Read the model definition and answer for the solid it produces. Units are mm, in the model's axes. A direction names the side the tool comes from. Round coordinates to 2 decimals unless told otherwise and drop trailing zeros. Answer as CSV lines item,"result".
```python
from build123d import *

# Parameters (mm, degrees)
SKETCH_1_R      = 11.25
SKETCH_1_R_2    = 1.5
SKETCH_1_W      = 5
SKETCH_1_H      = 10
EXTRUDE_1_DEPTH = 5


with BuildPart() as part:
    # 草图1 → 凸台-拉伸1 (new body)
    with BuildSketch(Plane(origin=(0, 0, 0), x_dir=(1, 0, 0), z_dir=(0, 1, 0))):
        Polygon((0, 0), (180, 0), (180, 5), (185, 5), (185, 15), (180, 15), (180, 19.659044965), (177.85, 19.659044965), (177.85, 18.15), (175.15, 18.15), (175.15, 19.659044965), (172, 19.659044965), (172, 22.65), (175.15, 22.65), (175.15, 24.15), (177.85, 24.15), (177.85, 22.65), (180, 22.65), (180, 27.3), (185, 27.3), (185, 37.3), (180, 37.3), (180, 42.3), (99, 42.3), (81, 42.3), (0, 42.3), (0, 37.3), (-5, 37.3), (-5, 27.3), (0, 27.3), (0, 22.65), (2.15, 22.65), (2.15, 24.15), (4.85, 24.15), (4.85, 22.65), (8, 22.65), (8, 19.659044965), (4.85, 19.659044965), (4.85, 18.15), (2.15, 18.15), (2.15, 19.659044965), (0, 19.659044965), (0, 15), (-5, 15), (-5, 5), (0, 5), align=None)
        with Locations(Location((65, 21.15, 0), (0, 0, 270))):
            Circle(SKETCH_1_R, mode=Mode.SUBTRACT)
        with Locations(Location((49.5, 36.65, 0), (0, 0, 270))):
            Circle(SKETCH_1_R_2, mode=Mode.SUBTRACT)
        with Locations(Location((80.5, 36.65, 0), (0, 0, 270))):
            Circle(SKETCH_1_R_2, mode=Mode.SUBTRACT)
        with Locations(Location((80.5, 5.65, 0), (0, 0, 270))):
            Circle(SKETCH_1_R_2, mode=Mode.SUBTRACT)
        with Locations(Location((49.5, 5.65, 0), (0, 0, 270))):
            Circle(SKETCH_1_R_2, mode=Mode.SUBTRACT)
        with Locations((37.5, 32.3)):
            Rectangle(SKETCH_1_W, SKETCH_1_H, mode=Mode.SUBTRACT)
        with Locations((37.5, 10)):
            Rectangle(SKETCH_1_W, SKETCH_1_H, mode=Mode.SUBTRACT)
        with Locations((142.5, 32.3)):
            Rectangle(SKETCH_1_W, SKETCH_1_H, mode=Mode.SUBTRACT)
        with Locations((142.5, 10)):
            Rectangle(SKETCH_1_W, SKETCH_1_H, mode=Mode.SUBTRACT)
    extrude(amount=EXTRUDE_1_DEPTH)


solid = part.part
```
Item 1: Flat-ended cylindrical pins translate along their axes: pin 1 (2.5 mm diameter, centred on x = 49.5, z = -5.65, fed in from -Y); pin 2 (1.7 mm diameter, centred on y = 3.5, z = -19, fed in from -X); pin 3 (1.6 mm diameter, centred on y = 1.5, z = -23.5, fed in from +X); pin 4 (1.5 mm diameter, centred on x = 183, y = 3, fed in from -Z). Find the tip coordinate at first contact, or state that the pin passes through.
Ans:
pin 1,"through"
pin 2,"x = 0"
pin 3,"x = 180"
pin 4,"z = -37.3"
Item 2: A cutting plane is placed at A-A, the plane y = 3.2. Give the number of separate pieces and of enclosed holes in the cut face, and give its area (3 significant figures).
Ans:
separate pieces,"1"
enclosed holes,"9"
area,"7,120 mm2"
Item 3: Determine the mould class of faces 1 (the face through (76.154, 2.465, -22.615)), 2 (the face through (182, 2, -27.3)), 3 (the face through (180, 2, -17)), 4 (the face through (48.036, 2.465, -5.975)) for opening direction X: +X half, -X half, draft (parallel to the pull), parting line (faces both ways), or undercut.
Ans:
face 1,"undercut"
face 2,"draft"
face 3,"+X half"
face 4,"undercut"
Item 4: A tool of negligible diameter and unlimited length cuts with its end or side. For faces 5 (the face through (-3, 2, -27.3)), 6 (the face through (174, 2, -19.659)), 7 (the face through (145, 2, -10)), 8 (the face through (-2, 2, -37.3)), from which of +Z, -Z, +X, -X, +Y, -Y can it reach the whole face along a straight path? Write none if from no direction.
Ans:
face 5,"-X, +Y, -Y"
face 6,"+X, +Y, -Y"
face 7,"+Y, -Y"
face 8,"-Z, -X, +Y, -Y"
Item 5: Find the intervals of material crossed by probe 1 along X at (y, z) = (1.15, -9.5); probe 2 along Z at (x, y) = (80.5, 3.5); probe 3 along X at (y, z) = (2.5, -5.65), in increasing order. Write a range as [from, to].
Ans:
probe 1,"[-5, 35], [40, 140], [145, 185]"
probe 2,"[-42.3, -38.15], [-35.15, -7.15], [-4.15, 0]"
probe 3,"[-5, 35], [40, 48], [51, 79], [82, 140], [145, 185]"
